Drawing for the job (mm, zero at the part's lowest x, y, z). A direction names the side the tool comes from. Give positions to 0.01 mm unless a question says otherwise; leave off trailing zeros. Write each loop counter-clockwise with the first axis right and the second up, starting at its lowest first coordinate (ties: lowest second). Pieces come first, ordered by that corner, then holes. Notation, with made-up numbers: (62.5, 19) - (71.5, 19) arc R9 ccw to (71.5, 34) - close; hole circle Ø3 at (6, -31.75). An arc over 180 degrees is marked (long way). Answer as a JSON object with one key per item and string values. Group by question number.
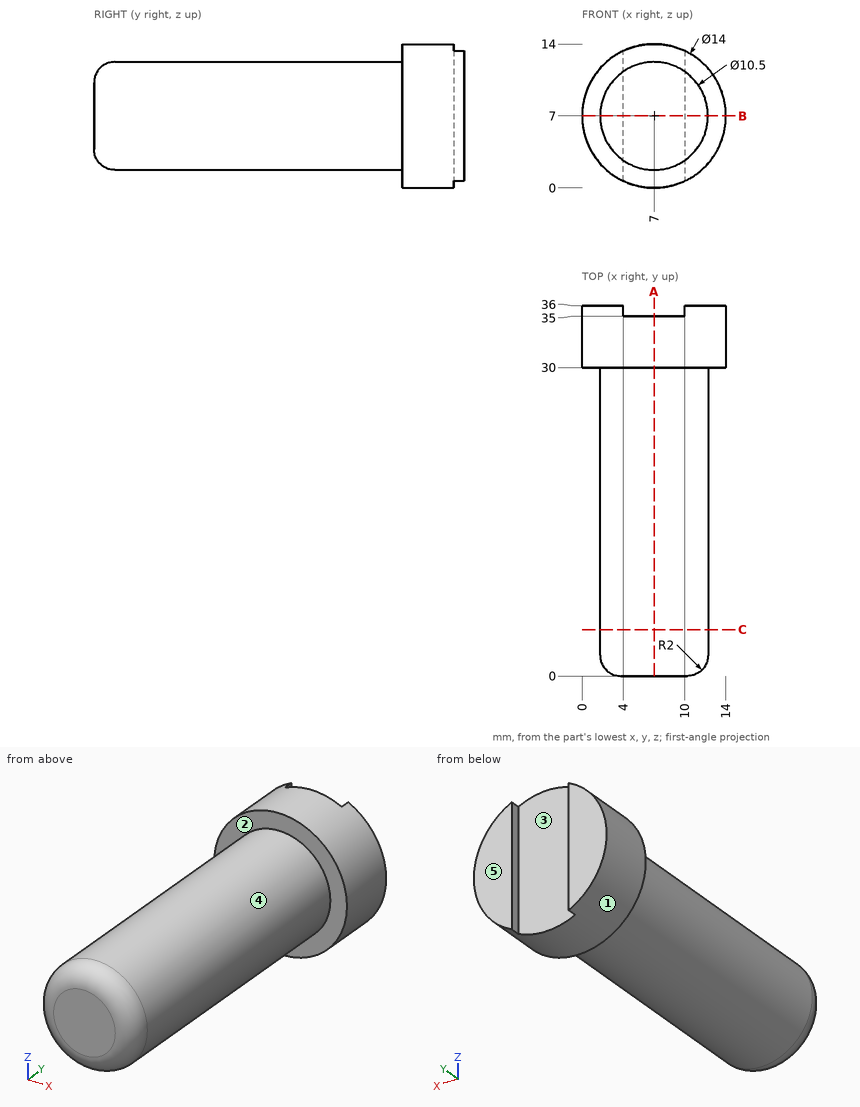
1) Band-saw the part on A-A (x = 7). List the corners of the cut face in (y, z).
2) Which spindle directions (+Z, -Z, +X, -X, +Y, -Y) get a long thin tool onto all of the face, cutting with end or side? Do the marked faces 1 and 2. Say none if no direction does.
3) Probe line 1 (Y direction, x = 6.75, z = 10.25); line 2 (Y direction, x = 13.25, z = 9); line 3 (Z direction, x = 6.75, y = 28). List the from-to ranges inside material, lowest first.
4) Mould opens along X. For the marked faces 3, 4 and 5 say: pulls with the +X half, pulls with the -X half, needs draft (parallel to the pull), parting line crosses it, or undercut.
5) Drop flat-ended pins along their axis: P1, Ø1.5, axis at x = 12, z = 2.5, coming from the -Y side; P2, Ø1, axis at x = 8.5, y = 24, coming from the -Z side; P3, Ø3, axis at y = 7, z = 8, coming from the -X side. Give the stop position or say it passes through.
6) Band-saw the part on C-C (y = 4.5). List the corners of the cut face in (x, z), plus the area to 3 significant figures.
7) Band-saw the part on B-B (z = 7). List the corners of the cut face in (x, y), plus the area to 3 significant figures.
Verdict:
{
 "1": {"outline": "(0, 3.75) arc R2 ccw to (2, 1.75) - (30, 1.75) - (30, 0) - (35, 0) - (35, 14) - (30, 14) - (30, 12.25) - (2, 12.25) arc R2 ccw to (0, 10.25) - close"},
 "2": {"face 1": "+Y, -Y", "face 2": "-Y"},
 "3": {"line 1": "0 to 35", "line 2": "30 to 36", "line 3": "1.76 to 12.24"},
 "4": {"face 3": "undercut", "face 4": "parting line crosses it", "face 5": "needs draft"},
 "5": {"P1": "y = 30", "P2": "z = 1.85", "P3": "x = 1.75"},
 "6": {"outline": "circle Ø10.5 at (7, 7)", "area": "86.6 mm2"},
 "7": {"outline": "(0, 30) - (1.75, 30) - (1.75, 2) arc R2 ccw to (3.75, 0) - (10.25, 0) arc R2 ccw to (12.25, 2) - (12.25, 30) - (14, 30) - (14, 36) - (10, 36) - (10, 35) - (4, 35) - (4, 36) - (0, 36) - close", "area": "391 mm2"}
}
